Build history of the part. All positions in model axes, mm. Round coordinates to 2 decimals unless told otherwise and drop trailing zeros. Loops run counter-clockwise (first coordinate to the right, second up) from the corner with the lowest first, then second, coordinate; pieces in that order, holes last. Notation, with made-up numbers: (85, 34.25) -> (95, 34.25) arc R18 cw to (95, 44.25) -> close; hole circle Ø6 at (-22, 5). An arc over 180 degrees is marked (long way). Put each result on its own line as item: value. Start each with the question number.
Autodesk Inventor part; units mm, degrees
ref_plane "YZ Plane" through (0, 0, 0) normal (1, 0, 0) x (0, 1, 0)
ref_plane "XZ Plane" through (0, 0, 0) normal (0, 1, 0) x (-1, 0, 0)
ref_plane "XY Plane" through (0, 0, 0) normal (0, 0, 1) x (1, 0, 0)
sketch "Sketch1" plane through (0, 0, 0) normal (0, 0, 1) x (1, 0, 0)
  line L0 (-25, 0) -> (25, 0)
  line L1 (25, 0) -> (25, -800)
  line L2 (25, -800) -> (-25, -800)
  line L3 (-25, -800) -> (-25, 0)
  point P0 (0, 0)
  point P1 (0, 0)
  dimension "d0" = 50
  dimension "d1" = 800
extrude "Plate1" add sketch "Sketch1" along normal blind 2
sketch "Sketch2" plane through (23, -800, 2) normal (1, 0, 0) x (0, 1, 0)
  line L0 (800, 0) -> (0, 0)
  line L1 (0, 0) -> (0, -30)
  line L2 (0, -30) -> (800, -30)
  line L3 (800, -30) -> (800, 0)
edge flange "Flange1" height 30 angle 90 thickness 2 bend radius 2.75 thickness toward (1, 0, 0) relief tear relief width 2 relief depth 1 corner gap 2 corner form 0 edges at (25, -400, 0) (-25, -400, 0) wall of the first edge with corners at (23, 0, 2) (23, -800, 2) (23, -800, -28) (23, 0, -28)
bend "Bend1"
corner "Corner1"
sketch "Sketch3" plane through (0, 0, 0) normal (1, 0, 0) x (0, 1, 0)
  line L0 (0, -2.75) -> (-800, -2.75)
  line L1 (-800, -28) -> (-800, -2.75)
  line L2 (0, -28) -> (-800, -28)
  line L3 (0, -2.75) -> (0, -28)
  line L4 (-790, -28) -> (-770, -28)
  line L5 (-770, -28) -> (-770, -18)
  line L6 (-770, -18) -> (-790, -18)
  line L7 (-790, -18) -> (-790, -28)
  point P0 (0, 0)
  point P1 (-770, -28)
  point P2 (-790, -23)
  dimension "d13" = 20
  dimension "d14" = 10
  dimension "d17" = 10
extrude "Extrusion1" [suppressed]
sketch "Sketch4" plane through (0, 0, 0) normal (0, 0, -1) x (-1, 0, 0)
  circle A0 centre (0, -733.4) radius 2.5
  circle A1 centre (0, -643.4) radius 2.5
  circle A2 centre (0, -155) radius 2.5
  circle A3 centre (0, -65) radius 2.5
  line L0 (20.25, 0) -> (-20.25, 0)
  line L1 (-20.25, 0) -> (20.25, 0)
  point P0 (0, 0)
  point P1 (0, 0)
  point P2 (0, 0)
  dimension "d18" = 5
  dimension "d19" = 90
  dimension "d20" = 90
  dimension "d21" = 488.4
  dimension "d22" = 65
extrude "Cut1" cut sketch "Sketch4" against normal blind 2
equation "\"d23\" = Thickness"
equation "\"d2\" = Thickness"
equation "\"d3\" = BendReliefWidth"
equation "\"d4\" = BendReliefDepth"
equation "\"d5\" = MinimumRemnant"
equation "\"d6\" = TransitionRadius"
equation "\"d10\" = CornerReliefSize"
equation "\"d11\" = GapSize"
equation "\"d12\" = JacobiRadiusSize"
equation "\"BendRadius\" = Thickness"
equation "\"BendReliefWidth\" = Thickness"
equation "\"BendReliefDepth\" = 0.5 * Thickness"
equation "\"CornerReliefSize\" = 4 * Thickness"
equation "\"MinimumRemnant\" = 2 * Thickness"
equation "\"TransitionRadius\" = BendRadius"
equation "\"JacobiRadiusSize\" = BendRadius"
equation "\"GapSize\" = Thickness"
properties part number "ДМФ 053 швеллер лотка v2.0_CPY"
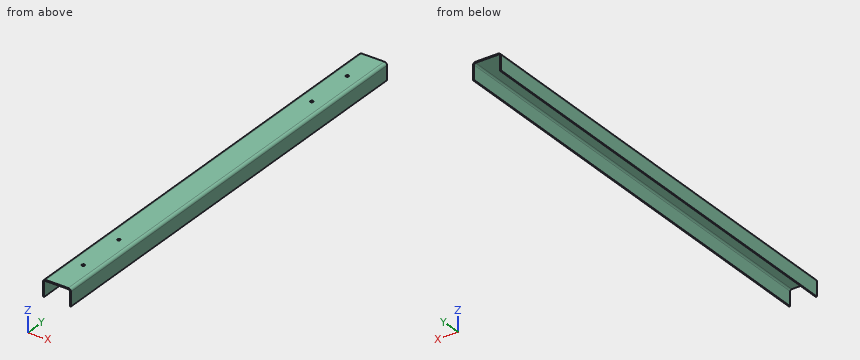
Item 1: Wall check: line 1 (Y direction, x = 0, z = 1.15); line 2 (X direction, y = -643.4, z = 1.1); line 3 (X direction, y = -56.5, z = -17). Give the ranges that are in metal, low to high. Write a range as from..to.
Item 2: Drop flat-ended pins along their axis: pin 1 (2 mm diameter, centred on y = -256, z = -1.5, fed in from -X); pin 2 (8 mm diameter, centred on x = 0, y = -155, fed in from +Z); pin 3 (20 mm diameter, centred on x = -6, y = -506.5, fed in from -Z). Give the stop position or say it passes through.
Item 3: Cut at C-C on x = -13.5. Write the cut outline in (y, z), then the cut area to 3 significant figures.
Item 4: Cut at B-B on y = -540. Write the cut outline in (x, z), then the cut area to 3 significant figures.
Item 5: Cut at A-A on z = -16. Write the cut outline in (x, y), then the cut area to 3 significant figures.
Ans:
1. line 1: y = -800..-735.9, -730.9..-645.9, -640.9..-157.5, -152.5..-67.5, -62.5..0
1. line 2: x = -23.03..-2.5, 2.5..23.03
1. line 3: x = -25..-23, 23..25
2. pin 1: stops at x = -24.99
2. pin 2: stops at z = 2
2. pin 3: stops at z = 0
3. outline: (-800, 0) -> (0, 0) -> (0, 2) -> (-800, 2) -> close
3. area: 1,600 mm2
4. outline: (-25, -28) -> (-23, -28) -> (-23, -2.75) arc R2.75 cw to (-20.25, 0) -> (20.25, 0) arc R2.75 cw to (23, -2.75) -> (23, -28) -> (25, -28) -> (25, -2.75) arc R4.75 ccw to (20.25, 2) -> (-20.25, 2) arc R4.75 ccw to (-25, -2.75) -> close
4. area: 206 mm2
5. outline: (-25, -800) -> (-23, -800) -> (-23, 0) -> (-25, 0) -> close; (23, -800) -> (25, -800) -> (25, 0) -> (23, 0) -> close
5. area: 3,200 mm2
